Can you work these out from the model? Positions are in its coordinate system, mm. Face numbers are marked on the shaded views. A direction names the side the tool comes from. Give positions to 0.01 mm unless a question says otherwise; leave off trailing zeros. Write each loop counter-clockwise with the first axis right and the second up, starting at its lowest first coordinate (ties: lowest second). Pieces come first, ordered by that corner, then holes.
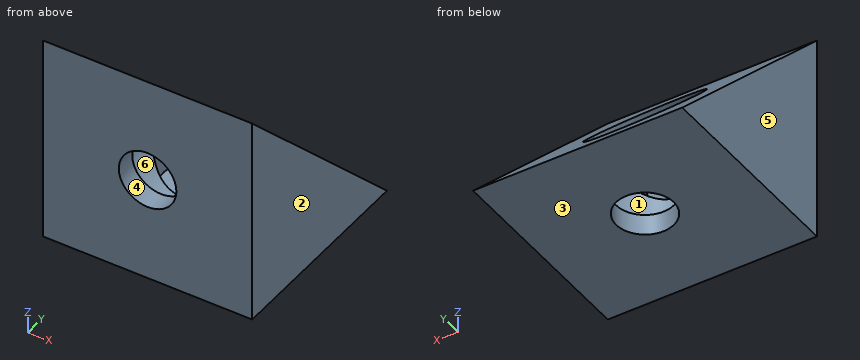
from build123d import *

# Parameters (mm, degrees)
CORNER_BASE_DEPTH      = 10
CORNER_BASE_DEPTH_BACK = 10
SKETCH2_R              = 2.75
SCREW_SHAFT_1_DEPTH    = 31
SKETCH3_R              = 2.75
SCREW_SHAFT_2_DEPTH    = 31
SKETCH4_R              = 5
SCREW_SOCKET_1_DEPTH   = 29.705400189
SKETCH5_R              = 5
CUT_EXTRUDE4_DEPTH     = 29.705400189


with BuildPart() as part:
    # Sketch1 → corner base (new, two sides: drawn at the far end of the back side and taken through both)
    with BuildSketch(Plane(origin=(0, 0, 0), x_dir=(0, 0, -1), z_dir=(1, 0, 0)).offset(-CORNER_BASE_DEPTH_BACK)):
        Polygon((0, 0), (0, 20), (-20, 0), align=None)
    extrude(amount=CORNER_BASE_DEPTH + CORNER_BASE_DEPTH_BACK)

    # Sketch2 → screw shaft 1 (cut, through all)
    with BuildSketch(Plane.XZ):
        with Locations(Location((0, 10, 0), (0, 0, 270))):
            Circle(SKETCH2_R)
    extrude(amount=-SCREW_SHAFT_1_DEPTH, mode=Mode.SUBTRACT)

    # Sketch3 → screw shaft 2 (cut, through all)
    with BuildSketch(Plane(origin=(0, 0, 0), x_dir=(-1, 0, 0), z_dir=(0, 0, -1))):
        with Locations((0, 10)):
            Circle(SKETCH3_R)
    extrude(amount=-SCREW_SHAFT_2_DEPTH, mode=Mode.SUBTRACT)

    # Sketch4 → screw socket 1 (cut, through all)
    with BuildSketch(Plane.XY.offset(2)):
        with Locations(Location((0, 10, 0), (0, 0, 90))):
            Circle(SKETCH4_R)
    extrude(amount=SCREW_SOCKET_1_DEPTH, mode=Mode.SUBTRACT)

    # Sketch5 → Cut-Extrude4 (cut, through all)
    with BuildSketch(Plane(origin=(0, 2, 0), x_dir=(1, 0, 0), z_dir=(0, 1, 0))):
        with Locations(Location((0, -10, 0), (0, 0, 180))):
            Circle(SKETCH5_R)
    extrude(amount=CUT_EXTRUDE4_DEPTH, mode=Mode.SUBTRACT)


solid = part.part
(1) For the marked faces 1 and 2, which set-ups out of +Z, -Z, +X, -X, +Y, -Y let a thin tool reach every point of the face, with its end or its side?
Returned:
face 1: +Z
face 2: +Z, -Z, +X, +Y, -Y
(2) Imagine slicing it at A-A, the plane z = 4. Write out the boundary of the cut face in (x, y), plus the area to 3 significant figures.
Returned:
outline: (-10, 0) - (10, 0) - (10, 16) - (-10, 16) - close; hole circle Ø10 at (0, 10)
area: 241 mm2
(3) Will these pins go through, and if not, where does the flat tip stop? P1, Ø9, axis at x = 0, z = 10, coming from the -Y side; P2, Ø2, axis at x = 5.5, y = 5, coming from the +Z side; P3, Ø8, axis at x = 0, y = 10, coming from the +Z side; P4, Ø8, axis at x = -1, z = 8, coming from the +Y side.
Returned:
P1: stops at y = 0
P2: stops at z = 16
P3: stops at z = 2
P4: stops at y = 16
(4) Imagine slicing it at D-D, the plane z = 9. Write out the boundary of the cut face in (x, y), plus the area to 3 significant figures.
Returned:
outline: (-10, 0) - (-2.56, 0) - (-2.56, 2) - (-4.9, 2) - (-4.9, 9) arc R5 cw to (-4.9, 11) - (-10, 11) - close; (2.56, 0) - (10, 0) - (10, 11) - (4.9, 11) arc R5 cw to (4.9, 9) - (4.9, 2) - (2.56, 2) - close
area: 121 mm2
(5) If I drill on L1, parallel to X at y = 0.75, z = 10; L2, parallel to Y at x = 6.5, z = 15; L3, parallel to X at y = 4.75, z = 6.5, over which ranges is the centre line in solid material (lowest first)?
Returned:
L1: x = -10 to -2.75, 2.75 to 10
L2: y = 0 to 5
L3: x = -10 to -3.57, 3.57 to 10
(6) Imagine slicing it at C-C, the plane y = 12.25. Write out the boundary of the cut face in (x, z).
Returned:
outline: (-10, 0) - (-1.58, 0) - (-1.58, 2) - (-4.47, 2) - (-4.47, 7.75) - (-10, 7.75) - close; (1.58, 0) - (10, 0) - (10, 7.75) - (4.47, 7.75) - (4.47, 2) - (1.58, 2) - close
(7) If we mould it in two halves opening along Z, with no side actions, what happens to the marked faces 3, 4, 5 and 6? For each: +Z half, -Z half, draft (parallel to the pull), parting line (faces both ways), or undercut.
Returned:
face 3: -Z half
face 4: undercut
face 5: draft
face 6: undercut
(8) Imagine slicing it at B-B, the plane x = 2.25. Write out the boundary of the cut face in (y, z), plus the area to 3 significant figures.
Returned:
outline: (0, 0) - (8.42, 0) - (8.42, 2) - (5.53, 2) - (5.53, 5.53) - (2, 5.53) - (2, 8.42) - (0, 8.42) - close; (0, 11.58) - (2, 11.58) - (2, 14.47) - (5.53, 14.47) - (0, 20) - close; (11.58, 0) - (20, 0) - (14.47, 5.53) - (14.47, 2) - (11.58, 2) - close
area: 84.3 mm2
